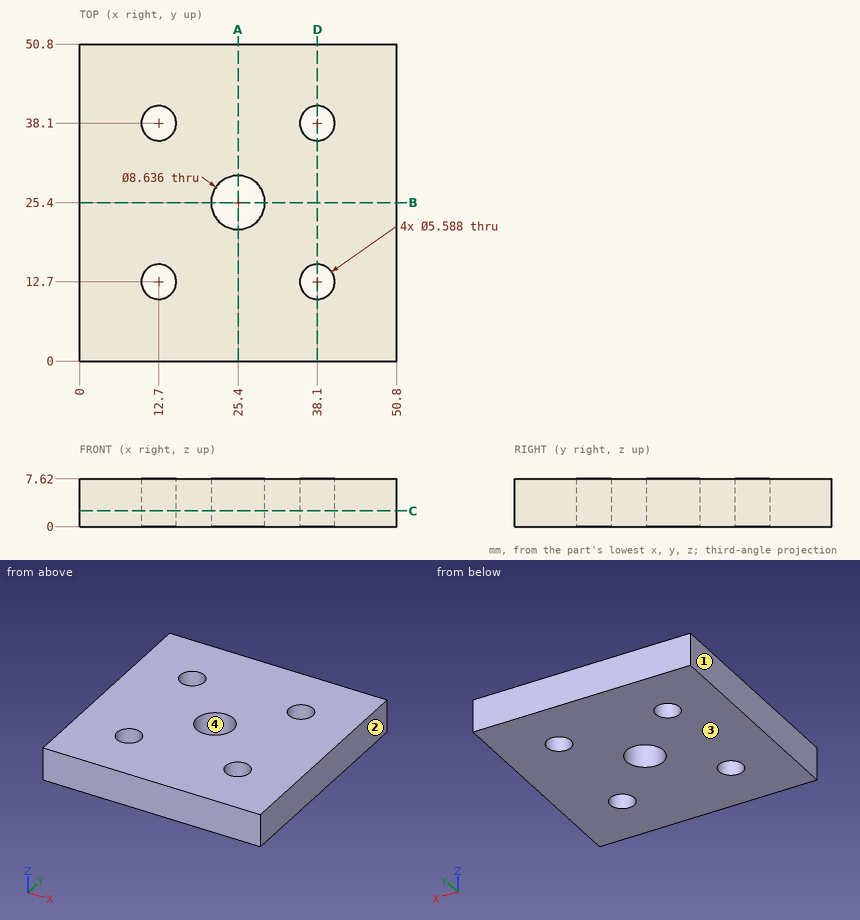
Geometry: see drawing. Coordinates: mm, zero at the bounding-box minimum. Give positions to 0.01 mm unless a question says otherwise; leave off trailing zeros. Write each loop counter-clockwise with the first axis right and the second up, starting at its lowest first coordinate (ties: lowest second). Pieces come first, ordered by that corner, then holes. Notation, with made-up numbers: (-4.5, 35.5) - (6.5, 35.5) arc R30 cw to (6.5, 66.5) - close; hole circle Ø5 at (6, 42). An arc over 180 degrees is marked (long way). Return JSON: item names as keys, results as strings. Group by question number.
1) Line query: line 1 (Y direction, x = 12.7, z = 5.75); line 2 (X direction, y = 14.5, z = 5); line 3 (Y direction, x = 36, z = 2.25). Output: solid intervals per line, ascending.
2) Mould query, pull axis X, two halves, no side actions, for the marked faces 1, 2, 3 and 4. Classes: released by +X, released by -X, zero draft, split by the parting line, or undercut.
3) Section A-A on x = 25.4. Return the cut outline in (y, z).
4) First-contact query: P1, Ø1.5, axis at y = 7.5, z = 2, coming from the -X side; P2, Ø5, axis at x = 38.1, y = 12.7, coming from the -Z side. Flat tips, straight axial feed; report the tip coordinate or a pass-through.
5) Section C-C on z = 2.5. Return the cut outline in (x, y), plus the area to 3 significant figures.
6) Section D-D on x = 38.1. Return the cut outline in (y, z), plus the area to 3 significant figures.
Filled in:
{
 "1": {"line 1": "y = 0 to 9.91, 15.49 to 35.31, 40.89 to 50.8", "line 2": "x = 0 to 10.56, 14.84 to 35.96, 40.24 to 50.8", "line 3": "y = 0 to 10.86, 14.54 to 36.26, 39.94 to 50.8"},
 "2": {"face 1": "released by -X", "face 2": "released by +X", "face 3": "zero draft", "face 4": "undercut"},
 "3": {"outline": "(0, 0) - (21.08, 0) - (21.08, 7.62) - (0, 7.62) - close; (29.72, 0) - (50.8, 0) - (50.8, 7.62) - (29.72, 7.62) - close"},
 "4": {"P1": "stops at x = 0", "P2": "passes through"},
 "5": {"outline": "(0, 0) - (50.8, 0) - (50.8, 50.8) - (0, 50.8) - close; hole circle Ø5.59 at (12.7, 12.7); hole circle Ø5.59 at (12.7, 38.1); hole circle Ø8.64 at (25.4, 25.4); hole circle Ø5.59 at (38.1, 12.7); hole circle Ø5.59 at (38.1, 38.1)", "area": "2,420 mm^2"},
 "6": {"outline": "(0, 0) - (9.91, 0) - (9.91, 7.62) - (0, 7.62) - close; (15.49, 0) - (35.31, 0) - (35.31, 7.62) - (15.49, 7.62) - close; (40.89, 0) - (50.8, 0) - (50.8, 7.62) - (40.89, 7.62) - close", "area": "302 mm^2"}
}
